from build123d import *

# Parameters (mm, degrees)
BOSS_EXTRUDE1_DEPTH = 10
SKETCH2_R           = 3.25
CUT_EXTRUDE1_DEPTH  = 6
SKETCH3_W           = 41
SKETCH3_H           = 23.5
SKETCH3_W_2         = 40
SKETCH3_H_2         = 22.5
BOSS_EXTRUDE3_DEPTH = 40
SKETCH4_W           = 7.997138399
SKETCH4_H           = 22.5
SKETCH4_W_2         = 8.001104186
BOSS_EXTRUDE4_DEPTH = 32
SKETCH5_R           = 1.261769867
SKETCH5_R_2         = 1.301986765
SKETCH5_R_3         = 1.319264735
SKETCH5_R_4         = 1.310040981
CUT_EXTRUDE2_DEPTH  = 6
FILLET1_R           = 2


with BuildPart() as part:
    # Sketch1 → Boss-Extrude1 (new body)
    with BuildSketch(Plane.XY):
        with BuildLine():
            Line((-63.656716418, 10.820895522), (66.343283582, 10.820895522))
            ThreePointArc((66.343283582, 10.820895522), (81.194029851, -4.029850746), (66.343283582, -18.880597015))
            Line((66.343283582, -18.880597015), (-63.656716418, -18.880597015))
            ThreePointArc((-63.656716418, -18.880597015), (-78.507462687, -4.029850746), (-63.656716418, 10.820895522))
        make_face()
    extrude(amount=BOSS_EXTRUDE1_DEPTH)

    # Sketch2 → Cut-Extrude1 (cut)
    with BuildSketch(Plane(origin=(0, 0, 0), x_dir=(-1, 0, 0), z_dir=(0, 0, -1))):
        with Locations((-66.343283582, -4.029850746)):
            Circle(SKETCH2_R)
    extrude(amount=-CUT_EXTRUDE1_DEPTH, mode=Mode.SUBTRACT)

    # Sketch3 → Boss-Extrude3 (add)
    with BuildSketch(Plane.XY.offset(10)):
        with Locations((-44.592304464, -3.554480068)):
            Rectangle(SKETCH3_W, SKETCH3_H)
        with Locations((-44.603010247, -3.550272792)):
            Rectangle(SKETCH3_W_2, SKETCH3_H_2, mode=Mode.SUBTRACT)
    extrude(amount=BOSS_EXTRUDE3_DEPTH)

    # Sketch4 → Boss-Extrude4 (add)
    with BuildSketch(Plane.XY.offset(10)):
        with Locations((-60.604441048, -3.550272792)):
            Rectangle(SKETCH4_W, SKETCH4_H)
        with Locations((-28.60356234, -3.550272792)):
            Rectangle(SKETCH4_W_2, SKETCH4_H)
    extrude(amount=BOSS_EXTRUDE4_DEPTH)

    # Sketch5 → Cut-Extrude2 (cut)
    with BuildSketch(Plane.XY.offset(42)):
        with Locations((-60.604441048, 3.806910367)):
            Circle(SKETCH5_R)
        with Locations((-28.60356234, 3.806910367)):
            Circle(SKETCH5_R_2)
        with Locations((-60.604441048, -11.471222054)):
            Circle(SKETCH5_R_3)
        with Locations((-28.60356234, -11.471222054)):
            Circle(SKETCH5_R_4)
    extrude(amount=-CUT_EXTRUDE2_DEPTH, mode=Mode.SUBTRACT)

    # Fillet1
    fillet1_edges = [part.edges().sort_by_distance(p)[0] for p in [
        (-65.092304464, -3.554480068, 10),
        (-44.592304464, -15.304480068, 10),
        (-24.092304464, -3.554480068, 10),
        (-44.592304464, 8.195519932, 10),
        (-44.60499314, 7.699727208, 10),
    ]]
    fillet(fillet1_edges, radius=FILLET1_R)


solid = part.part
For this review, take the finished solid that the model builds, in its own axes (mm). A direction names the side the tool comes from. Round coordinates to 2 decimals unless told otherwise and drop trailing zeros. Write each loop counter-clockwise with the first axis right and the second up, starting at its lowest first coordinate (ties: lowest second). Pieces come first, ordered by that corner, then holes. Notation, with made-up numbers: M -20.75,2.5 L 16.25,2.5 A21 ccw 16.25,6.5 Z; hole C -27.5,-19 d7. An arc over 180 degrees is marked long. Write item = value, one per line. Start each with the question number.
(1) For faces 1 (the face through (-65.092, -4, 31)), 2 (the face through (-29, -11, 36)), 3 (the face through (-78.504, -4.356, 4.93)), list the 3-axis set-ups (+Z, -Z, +X, -X, +Y, -Y) from which the entire face can be reached by the end or side of a thin tool; tool diameter is ignored.
(2) We need section C-C (x = 30). Give the boundary of the cut face in (y, z), then the cut area to 3 significant figures.
(3) Clearance check with flat-ended pins moving along their axes: pin 1 Ø2 at (x, y) = (-28.5, 4) entering from +Z; pin 2 Ø6 at (y, z) = (6.5, 27.5) entering from +X; pin 3 Ø6 at (y, z) = (-6.5, 32) entering from -X. State where each tip first meets the part, or that it passes through.
(4) We need section B-B (x = -39.5). Give the boundary of the cut face in (y, z), then the cut area to 3 significant figures.
(5) We need section A-A (z = 19). Give the boundary of the cut face in (x, y), then the cut area to 3 significant figures.
(6) For line 1 along X through (y, z) = (-1.25, 39); line 2 along X through (y, z) = (-14, 43); line 3 along Y through (x, z) = (-49.5, 48), list the stretches that pass through material, from the lowest coordinate up.
(7) The part is to be moulded in two halves that separate along X. For faces 4 (the face through (-24.092, -4, 31)), 5 (the face through (-32.604, -4, 26)), 6 (the face through (-45, 8.196, 31)), say which applies: +X half, -X half, draft (parallel to the pull), parting line (faces both ways), or undercut.
Results found:
q1.face_1 = +Z, -X, +Y, -Y
q1.face_2 = +Z
q1.face_3 = +Z, -Z, -X
q2.outline = M -18.88,0 L 10.82,0 L 10.82,10 L -18.88,10 Z
q2.area = 297 mm²
q3.pin_1 = 36
q3.pin_2 = -24.09
q3.pin_3 = -65.09
q4.outline = M -18.88,0 L 10.82,0 L 10.82,10 L 10.2,10 A2 cw 8.2,12 L 8.2,50 L 7.7,50 L 7.7,12 A2 cw 5.7,10 L -14.8,10 L -14.8,50 L -15.3,50 L -15.3,12 A2 cw -17.3,10 L -18.88,10 Z
q4.area = 340 mm²
q5.outline = M -65.09,-15.3 L -24.09,-15.3 L -24.09,8.2 L -65.09,8.2 Z; hole M -56.61,-14.8 L -32.6,-14.8 L -32.6,7.7 L -56.61,7.7 Z
q5.area = 423 mm²
q6.line_1 = -65.09 to -56.61, -32.6 to -24.09
q6.line_2 = -65.09 to -64.6, -24.6 to -24.09
q6.line_3 = -15.3 to -14.8, 7.7 to 8.2
q7.face_4 = +X half
q7.face_5 = undercut
q7.face_6 = draft
